The model under review builds one solid part; all positions refer to its coordinate system, in mm. Face numbers are marked on the shaded views. A direction names the side the tool comes from. Round coordinates to 2 decimals unless told otherwise and drop trailing zeros. Order: outer loops, then holes, each group sorted by start corner. A loop starts at its lowest first (then second) coordinate and runs counter-clockwise, first axis right, second up.
1) To check wall thickness, follow L1, parallel to Y at x = 14.25, z = -21; L2, parallel to Y at x = -4, z = -14; L3, parallel to Y at x = 16, z = -7.25. State the ranges of each line that lie inside material, in increasing order.
2) Consider section A-A (y = 0). Give the boundary of the cut face in (x, z), then the cut area to 3 significant figures.
3) Consider section C-C (z = -14). Give the boundary of the cut face in (x, y).
4) Machinability: for the marked faces 1 and 2, which of the approach directions +Z, -Z, +X, -X, +Y, -Y give a long, thin tool a straight path to every point of the face, cutting with its end or side? Answer none if there is none.
5) Consider section D-D (y = -14.25). Give the number of separate pieces and of enclosed holes in the cut face, then the cut area to 3 significant figures.
6) Clearance check with flat-ended pins moving along their axes: P1, Ø6, axis at x = -32.5, z = -17.5, coming from the +Y side; P2, Ø1, axis at y = -24.5, z = -22.5, coming from the +X side; P3, Ø4, axis at y = 27.5, z = -16, coming from the -X side; P4, Ø1.5, axis at x = 13, z = -22.5, coming from the -Y side. State where each tip first meets the part, or that it passes through.
from build123d import *

# Parameters (mm, degrees)
SKETCH2_R          = 2
CUT_EXTRUDE1_DEPTH = 72.637978754


with BuildPart() as part:
    # Sketch1 → Revolve1 (revolve)
    with BuildSketch(Plane(origin=(0, 0, 0), x_dir=(0, 0, -1), z_dir=(1, 0, 0)), mode=Mode.PRIVATE) as revolve1_sk:
        Polygon((0, 10), (0, 27.5), (5, 46), (6.5, 46), (1.5, 27.5), (30, 27.5), (30, 10), align=None)
    revolve(revolve1_sk.sketch.rotate(Axis((0, 0, 467.574650711), (0, 0, -1)), 90), axis=Axis((0, 0, 467.574650711), (0, 0, -1)))

    # Sketch2 → Cut-Extrude1 (cut, through all)
    with BuildSketch(Plane.XY):
        with Locations((-14.25, 14.25)):
            Circle(SKETCH2_R)
        with Locations((14.25, 14.25)):
            Circle(SKETCH2_R)
        with Locations((14.25, -14.25)):
            Circle(SKETCH2_R)
        with Locations((-14.25, -14.25)):
            Circle(SKETCH2_R)
    extrude(amount=-CUT_EXTRUDE1_DEPTH, mode=Mode.SUBTRACT)


solid = part.part
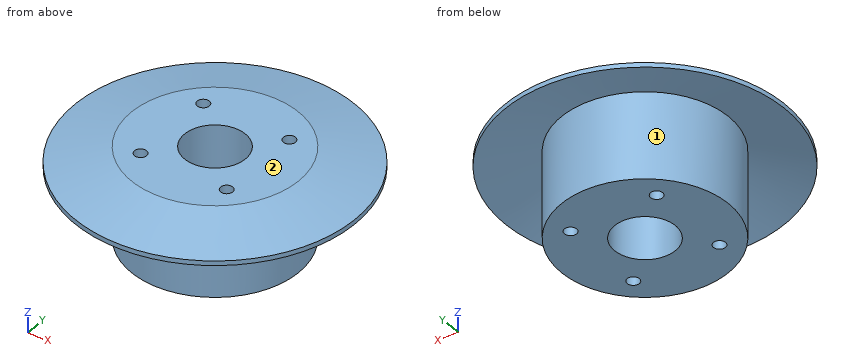
Answer below:
1. L1: y = -23.52 to -16.25, -12.25 to 12.25, 16.25 to 23.52
1. L2: y = -27.21 to -9.17, 9.17 to 27.21
1. L3: y = -22.37 to -15.22, -13.28 to 13.28, 15.22 to 22.37
2. outline: (-46, -6.5) - (-27.5, -1.5) - (-27.5, -30) - (-10, -30) - (-10, 0) - (-27.5, 0) - (-46, -5) - close; (10, -30) - (27.5, -30) - (27.5, -1.5) - (46, -6.5) - (46, -5) - (27.5, 0) - (10, 0) - close
2. area: 1,110 mm2
3. outline: circle Ø55 at (0, 0); hole circle Ø4 at (-14.25, -14.25); hole circle Ø4 at (-14.25, 14.25); hole circle Ø20 at (0, 0); hole circle Ø4 at (14.25, -14.25); hole circle Ø4 at (14.25, 14.25)
4. face 1: -Z
4. face 2: +Z, +X, -X, +Y, -Y
5. separate pieces: 3
5. enclosed holes: 0
5. area: 1,230 mm2
6. P1: passes through
6. P2: stops at x = 13.43
6. P3: stops at x = -10.3
6. P4: stops at y = -24.62
